```python
from build123d import *


with BuildPart() as part:
    # Croquis1 → Revolución1 (revolve)
    with BuildSketch(Plane.XY, mode=Mode.PRIVATE) as revoluci_n1_sk:
        Polygon((0, 0), (0, 16.40097141), (35, 16.40097141), (35, 38.90097141), (70, 38.90097141), (70, 60.089754962), (105, 60.089754962), (105, 48.950400909), (88, 48.950400909), (88, 28.083723598), (58, 28.083723598), (58, 10.791148393), (75, 10.791148393), (75, 0), align=None)
    revolve(revoluci_n1_sk.sketch.rotate(Axis((0, -38.59902859, 0), (1, 0, 0)), 90), axis=Axis((0, -38.59902859, 0), (1, 0, 0)))


solid = part.part
```
For this review, take the finished solid that the model builds, in its own axes (mm). A direction names the side the tool comes from. Round coordinates to 2 decimals unless told otherwise and drop trailing zeros. Write each loop counter-clockwise with the first axis right and the second up, starting at its lowest first coordinate (ties: lowest second). Pieces come first, ordered by that corner, then holes.
1) For line 1 along Y through (x, z) = (73, 0); line 2 along Y through (x, z) = (81.25, 0); line 3 along Z through (x, y) = (72, -47), list the stretches that pass through material, from the lowest coordinate up.
Answer below:
line 1: y = -137.29 to -105.28, -87.99 to -77.2, 0 to 10.79, 28.08 to 60.09
line 2: y = -137.29 to -105.28, 28.08 to 60.09
line 3: z = -98.33 to -66.15, -48.67 to -37.67, 37.67 to 48.67, 66.15 to 98.33
2) Take a section at D-D on y = 7. Give the boundary of the cut face in (x, z), then the cut area to 3 significant figures.
Answer below:
outline: (0, -30.75) - (35, -30.75) - (35, -62.67) - (70, -62.67) - (70, -87.52) - (105, -87.52) - (105, -74.74) - (88, -74.74) - (88, -48.66) - (58, -48.66) - (58, -18.98) - (75, -18.98) - (75, 18.98) - (58, 18.98) - (58, 48.66) - (88, 48.66) - (88, 74.74) - (105, 74.74) - (105, 87.52) - (70, 87.52) - (70, 62.67) - (35, 62.67) - (35, 30.75) - (0, 30.75) - close
area: 7,850 mm2
3) Take a section at C-C on x = 85. Give the boundary of the cut face in (y, z).
Answer below:
outline: circle Ø197.38 at (-38.6, 0); hole circle Ø133.37 at (-38.6, 0)
4) Take a section at B-B on y = -61. Give the boundary of the cut face in (x, z).
Answer below:
outline: (0, -50.23) - (35, -50.23) - (35, -74.19) - (70, -74.19) - (70, -96.11) - (105, -96.11) - (105, -84.64) - (88, -84.64) - (88, -62.81) - (58, -62.81) - (58, -44.02) - (75, -44.02) - (75, -31.43) - (0, -31.43) - close; (0, 31.43) - (75, 31.43) - (75, 44.02) - (58, 44.02) - (58, 62.81) - (88, 62.81) - (88, 84.64) - (105, 84.64) - (105, 96.11) - (70, 96.11) - (70, 74.19) - (35, 74.19) - (35, 50.23) - (0, 50.23) - close
5) Insertion check: pin 1 Ø1.5 at (x, z) = (14.5, 3.5) entering from -Y; pin 2 Ø1.5 at (x, z) = (45, 34) entering from -Y; pin 3 Ø4 at (x, y) = (12.5, -33.5) entering from -Z. Each pin has a flat end and moves straight along its axis. Give the tip position at first contact, or say it passes through.
Answer below:
pin 1: stops at y = -93.53
pin 2: stops at y = -108.6
pin 3: stops at z = -54.91
6) Machinability: for faces 1 (the face through (0, -76, -11)), 2 (the face through (58, -39, -50)), 3 (the face through (17.74, -93.13, -7.16)), which of the approach directions +Z, -Z, +X, -X, +Y, -Y give a long, thin tool a straight path to every point of the face, cutting with its end or side? Answer none if there is none.
Answer below:
face 1: +Z, -Z, -X, +Y, -Y
face 2: +X
face 3: -X
7) Mouldability with a two-part tool opening along Z and no side actions: class faces 4 (the face through (87.745, 21.452, -78.316)), 5 (the face through (105, 41, -37)), 6 (the face through (96.38, 46.87, -18.98)) as +Z half, -Z half, draft (parallel to the pull), parting line (faces both ways), or undercut.
Answer below:
face 4: parting line
face 5: draft
face 6: undercut
8) Take a section at A-A on z = 0. Give the boundary of the cut face in (x, y), then the cut area to 3 significant figures.
Answer below:
outline: (0, -93.6) - (35, -93.6) - (35, -116.1) - (70, -116.1) - (70, -137.29) - (105, -137.29) - (105, -126.15) - (88, -126.15) - (88, -105.28) - (58, -105.28) - (58, -87.99) - (75, -87.99) - (75, -77.2) - (0, -77.2) - close; (0, 0) - (75, 0) - (75, 10.79) - (58, 10.79) - (58, 28.08) - (88, 28.08) - (88, 48.95) - (105, 48.95) - (105, 60.09) - (70, 60.09) - (70, 38.9) - (35, 38.9) - (35, 16.4) - (0, 16.4) - close
area: 5,090 mm2
